Verification items for the finished model (mm, model axes). Face numbers are marked on the shaded views. A direction names the side the tool comes from. Round coordinates to 2 decimals unless told otherwise and drop trailing zeros. Write each loop counter-clockwise with the first axis right and the second up, starting at its lowest first coordinate (ties: lowest second). Pieces come first, ordered by that corner, then holes. Notation, with made-up numbers: (34.25, -16.75) - (41.25, -16.75) arc R24 ccw to (41.25, 3.25) - close; hole circle Ø9 at (82.25, 18.25). An arc over 180 degrees is marked (long way). Answer as a JSON object with one key per item and string values.
```python
from build123d import *

# Parameters (mm, degrees)
SKETCH_1_W          = 94
SKETCH_1_H          = 28
SKETCH_1_R          = 2
SKETCH_1_H_2        = 30
SKETCH_1_R_2        = 2.6
EXTRUDE_1_DEPTH     = 5
SKETCH_2_W          = 20
SKETCH_2_H          = 10
SKETCH_2_H_2        = 9.9565682
SKETCH_2_H_3        = 9.91450181
CUT_EXTRUDE_1_DEPTH = 3.8
SKETCH_3_W          = 18
SKETCH_3_H          = 10
CUT_EXTRUDE_2_DEPTH = 0.8
SKETCH_4_W          = 0.5
SKETCH_4_H          = 10
CUT_EXTRUDE_3_DEPTH = 6


with BuildPart() as part:
    # 草图1 → 凸台-拉伸1 (new body)
    with BuildSketch(Plane.XY):
        with Locations((46.493576546, 13.050650803)):
            Rectangle(SKETCH_1_W, SKETCH_1_H)
        with Locations((11.243576546, 19.050650803)):
            Circle(SKETCH_1_R, mode=Mode.SUBTRACT)
        with Locations((34.743576546, 19.007901708)):
            Circle(SKETCH_1_R, mode=Mode.SUBTRACT)
        with Locations((58.243576546, 19.028934903)):
            Circle(SKETCH_1_R, mode=Mode.SUBTRACT)
        with Locations((81.743576546, 19.050650803)):
            Circle(SKETCH_1_R, mode=Mode.SUBTRACT)
        with Locations((46.493576546, -15.949349197)):
            Rectangle(SKETCH_1_W, SKETCH_1_H_2)
        with Locations((14.493576546, -15.949349197)):
            Circle(SKETCH_1_R_2, mode=Mode.SUBTRACT)
        with Locations((78.493576546, -15.949349197)):
            Circle(SKETCH_1_R_2, mode=Mode.SUBTRACT)
    extrude(amount=EXTRUDE_1_DEPTH)

    # 草图2 → 切除-拉伸1 (cut)
    with BuildSketch(Plane(origin=(0, 0, 0), x_dir=(-1, 0, 0), z_dir=(0, 0, -1))):
        with Locations((-81.743576546, 19.050650803)):
            Rectangle(SKETCH_2_W, SKETCH_2_H)
        with Locations((-58.243576546, 19.028934903)):
            Rectangle(SKETCH_2_W, SKETCH_2_H_2)
        with Locations((-34.743576546, 19.007901708)):
            Rectangle(SKETCH_2_W, SKETCH_2_H_3)
        with Locations((-11.243576546, 19.050650803)):
            Rectangle(SKETCH_2_W, SKETCH_2_H)
    extrude(amount=-CUT_EXTRUDE_1_DEPTH, mode=Mode.SUBTRACT)

    # 草图3 → 切除-拉伸2 (cut)
    with BuildSketch(Plane(origin=(0, 0, 0), x_dir=(-1, 0, 0), z_dir=(0, 0, -1))):
        with Locations((-4.493576546, 6.550650803)):
            Rectangle(SKETCH_3_W, SKETCH_3_H)
        with Locations((-27.993576546, 6.550650803)):
            Rectangle(SKETCH_3_W, SKETCH_3_H)
        with Locations((-51.493576546, 6.550650803)):
            Rectangle(SKETCH_3_W, SKETCH_3_H)
        with Locations((-74.993576546, 6.550650803)):
            Rectangle(SKETCH_3_W, SKETCH_3_H)
        with Locations((-98.493576546, 6.550650803)):
            Rectangle(SKETCH_3_W, SKETCH_3_H)
    extrude(amount=-CUT_EXTRUDE_2_DEPTH, mode=Mode.SUBTRACT)

    # 草图4 → 切除-拉伸3 (cut, through all)
    with BuildSketch(Plane(origin=(0, 0, 0), x_dir=(-1, 0, 0), z_dir=(0, 0, -1))):
        with Locations((-13.243576546, 6.550650803)):
            Rectangle(SKETCH_4_W, SKETCH_4_H)
        with Locations((-19.243576546, 6.550650803)):
            Rectangle(SKETCH_4_W, SKETCH_4_H)
        with Locations((-36.743576546, 6.550650803)):
            Rectangle(SKETCH_4_W, SKETCH_4_H)
        with Locations((-42.743576546, 6.550650803)):
            Rectangle(SKETCH_4_W, SKETCH_4_H)
        with Locations((-60.243576546, 6.550650803)):
            Rectangle(SKETCH_4_W, SKETCH_4_H)
        with Locations((-66.243576546, 6.550650803)):
            Rectangle(SKETCH_4_W, SKETCH_4_H)
        with Locations((-83.743576546, 6.550650803)):
            Rectangle(SKETCH_4_W, SKETCH_4_H)
        with Locations((-89.743576546, 6.550650803)):
            Rectangle(SKETCH_4_W, SKETCH_4_H)
    extrude(amount=-CUT_EXTRUDE_3_DEPTH, mode=Mode.SUBTRACT)


solid = part.part
```
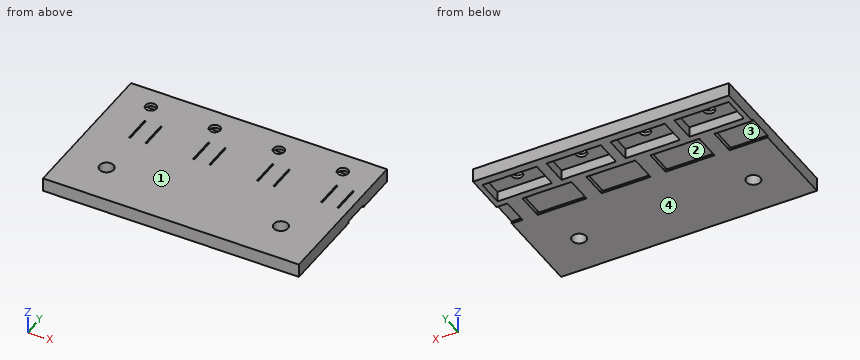
Q1. Section check C-C, the plane y = -17. Record the cut outline in (x, z).
Geometry check:
{"outline": "(-0.51, 0) - (12.12, 0) - (12.12, 5) - (-0.51, 5) - close; (16.87, 0) - (76.12, 0) - (76.12, 5) - (16.87, 5) - close; (80.87, 0) - (93.49, 0) - (93.49, 5) - (80.87, 5) - close"}
Q2. Section check D-D, the plane y = 9.5. State how many separate pieces and enclosed holes the cut face has, then the cut area to 3 significant figures.
Geometry check:
{"separate pieces": "9", "enclosed holes": "0", "area": "396 mm2"}
Q3. Material ranges on line 1 along X through (y, z) = (5, 0.7); line 2 along X through (y, z) = (18, 1.65); line 3 along Y through (x, z) = (53, 3.15), recorded low to high. Write a range as [from, to].
Geometry check:
{"line 1": "x = [13.49, 18.99], [36.99, 42.49], [60.49, 65.99], [83.99, 89.49]", "line 2": "x = [-0.51, 1.24], [21.24, 24.74], [44.74, 48.24], [68.24, 71.74], [91.74, 93.49]", "line 3": "y = [-30.95, 14.05], [24.01, 27.05]"}
Q4. Section check A-A, the plane x = 10.5. Record the cut outline in (y, z).
Geometry check:
{"outline": "(-30.95, 0) - (1.55, 0) - (1.55, 0.8) - (11.55, 0.8) - (11.55, 0) - (14.05, 0) - (14.05, 3.8) - (17.19, 3.8) - (17.19, 5) - (-30.95, 5) - close; (20.91, 3.8) - (24.05, 3.8) - (24.05, 0) - (27.05, 0) - (27.05, 5) - (20.91, 5) - close"}
Q5. Gauge pin test, flat ends, axial feed: P1, Ø3, axis at x = 74.5, y = 7.5, coming from the -Z side; P2, Ø5, axis at x = 81.74, y = 19.05, coming from the -Z side; P3, Ø10, axis at x = 74, y = -4.5, coming from the -Z side. Record the tip position at first contact, or that the pin passes through.
Geometry check:
{"P1": "stops at z = 0.8", "P2": "stops at z = 3.8", "P3": "stops at z = 0"}
Q6. Set-up check for the marked faces 1 and 2: record each of +Z, -Z, +X, -X, +Y, -Y from which the full face is reachable in a straight line by a thin tool's end or side.
Geometry check:
{"face 1": "+Z, +X, -X, +Y, -Y", "face 2": "-Z"}
Q7. Release check for a two-part mould opening along Y. For the marked faces 3 and 4 record: released by +Y, released by -Y, zero draft, split by the parting line, or undercut.
Geometry check:
{"face 3": "undercut", "face 4": "zero draft"}
Q8. Section check B-B, the plane x = 65. Record the cut outline in (y, z), then the cut area to 3 significant figures.
Geometry check:
{"outline": "(-30.95, 0) - (14.05, 0) - (14.05, 3.8) - (24.01, 3.8) - (24.01, 0) - (27.05, 0) - (27.05, 5) - (-30.95, 5) - close", "area": "252 mm2"}
